Build history of the part. All positions in model axes, mm. A direction names the side the tool comes from. Coordinates: 2 decimals unless noted, no trailing zeros. Loops run counter-clockwise (first coordinate to the right, second up) from the corner with the lowest first, then second, coordinate; pieces in that order, holes last. Notation, with made-up numbers: M -8.75,41 L 1.25,41 A9 ccw 1.25,52 Z; hole C 18,-18 d7. An arc over 180 degrees is marked long. Write each question's results on one line, items separated by ' | '. Start each with the question number.
from build123d import *

# Parameters (mm, degrees)
F0_W     = 12.7
F0_H     = 19.05
F1_DEPTH = 76.2
F3_DEPTH = 25.4
F4_D     = 5.1054
F5_R     = 1.524


with BuildPart() as f1:
    # F0 (on Right) → F1 (new body)
    with BuildSketch(Plane.YZ):
        with Locations((6.35, 9.525)):
            Rectangle(F0_W, F0_H)
    extrude(amount=F1_DEPTH)

    # F2 (on face) → F3 (cut)
    with BuildSketch(Plane.XZ):
        with BuildLine():
            Line((6.35, 9.398), (3.1623, 9.398))
            ThreePointArc((3.1623, 9.398), (6.35, 6.2103), (9.5377, 9.398))
            Line((9.5377, 9.398), (6.35, 9.398))
        make_face()
        with BuildLine():
            Line((66.6623, 9.398), (65.8400815402, 0))
            Line((65.8400815402, 0), (73.0377, 0))
            Line((73.0377, 0), (73.0377, 9.398))
            ThreePointArc((73.0377, 9.398), (69.85, 12.5857), (66.6623, 9.398))
        make_face()
        with BuildLine():
            ThreePointArc((9.5377, 9.398), (6.35, 12.5857), (3.1623, 9.398))
            Line((3.1623, 9.398), (6.35, 9.398))
            Line((6.35, 9.398), (9.5377, 9.398))
        make_face()
    extrude(amount=-F3_DEPTH, mode=Mode.SUBTRACT)

    # F4 (through all)
    with Locations(Plane.XZ):
        with Locations((38.1, 9.398)):
            Hole(F4_D / 2)

    # F5
    f5_edges = [f1.edges().sort_by_distance(p)[0] for p in [
        (76.2, 6.35, 19.05),
        (0, 6.35, 19.05),
        (76.2, 6.35, 0),
        (0, 6.35, 0),
    ]]
    fillet(f5_edges, radius=F5_R)


solid = f1.part
1. Band-saw the part on B-B, the plane y = 3. List the corners of the cut face in (x, z).
2. Wall check: line 1 along X through (y, z) = (4.25, 11); line 2 along X through (y, z) = (11.75, 8.75); line 3 along Z through (x, y) = (38.1, 4). Give the ranges that are in metal, low to high.
3. Mould opens along Z. For faces 3 (the flat face through (76.2, 6, 10)), 4 (the cylindrical face through (7.82, 6.26, 6.57)), 5 (the flat face through (74, 6, 0)) say: +Z half, -Z half, draft (parallel to the pull), parting line (faces both ways), or undercut.
4. Band-saw the part on A-A, the plane x = 38.1. List the corners of the cut face in (y, z), plus the area to 3 significant figures.
5. Band-saw the part on D-D, the plane x = 69.85. List the corners of the cut face in (y, z), plus the area to 3 significant figures.
6. Band-saw the part on C-C, the plane x = 6.35. List the corners of the cut face in (y, z), plus the area to 3 significant figures.
7. Which spindle directions (+Z, -Z, +X, -X, +Y, -Y) get a long thin tool onto all of the face, cutting with end or side? Do faces 1 (the flat face through (66.257, 6.261, 4.765)), 2 (the flat face through (38, 12.7, 14)). Say none if no direction does.
8. Pin check, flat tip, straight feed: pin 1 (3 mm diameter, centred on x = 38.1, z = 9.398, fed in from +Y). Stop position of the tip, or through.
Checked values:
1) outline: M 0,1.52 A1.52 ccw 1.52,0 L 65.84,0 L 66.66,9.4 A3.19 cw 73.04,9.4 L 73.04,0 L 74.68,0 A1.52 ccw 76.2,1.52 L 76.2,17.53 A1.52 ccw 74.68,19.05 L 1.52,19.05 A1.52 ccw 0,17.53 Z; hole C 6.35,9.4 d6.38; hole C 38.1,9.4 d5.11
2) line 1: 0 to 3.59, 9.11 to 36.11, 40.09 to 67.09, 72.61 to 76.2 | line 2: 0 to 3.23, 9.47 to 35.63, 40.57 to 66.61, 73.04 to 76.2 | line 3: 0 to 6.85, 11.95 to 19.05
3) face 3: draft | face 4: undercut | face 5: -Z half
4) outline: M 0,0 L 12.7,0 L 12.7,6.85 L 0,6.85 Z; M 0,11.95 L 12.7,11.95 L 12.7,19.05 L 0,19.05 Z | area: 177 mm²
5) outline: M 0,12.59 L 12.7,12.59 L 12.7,19.05 L 0,19.05 Z | area: 82.1 mm²
6) outline: M 0,0 L 12.7,0 L 12.7,6.21 L 0,6.21 Z; M 0,12.59 L 12.7,12.59 L 12.7,19.05 L 0,19.05 Z | area: 161 mm²
7) face 1: -Z, +Y, -Y | face 2: +Z, -Z, +X, -X, +Y
8) pin 1: through
